Job drawing, mm, ordinate dimensions from the low corner. One solid piece. A direction names the side the tool comes from. Round coordinates to 2 decimals unless told otherwise and drop trailing zeros. Write each loop counter-clockwise with the first axis right and the second up, starting at its lowest first coordinate (ties: lowest second). Pieces come first, ordered by that corner, then holes.
1) Saw through at A-A (y = 180). Write the cut outline in (x, z), plus the area to 3 significant figures.
2) Which spindle directions (+Z, -Z, +X, -X, +Y, -Y) get a long thin tool onto all of the face, cutting with end or side? Do the marked faces 4, 5, 6 and 7. Say none if no direction does.
3) Saw through at B-B (z = 30). Write the cut outline in (x, y).
4) Saw through at D-D (z = 54). Write the cut outline in (x, y).
5) Wall check: probe 1 along Y at (x, z) = (17, 30); probe 2 along Y at (x, z) = (24, 30); probe 3 along Y at (x, z) = (42, 11). Give the ranges that are in metal, low to high.
6) Flat gauge pins, fed straight in: pin 1 (12.5 mm diameter, centred on x = 33.5, y = 165.5, fed in from +Z); pin 2 (8 mm diameter, centred on y = 51, z = 24, fed in from +X); pin 3 (1.5 mm diameter, centred on x = 47.5, z = 8, fed in from +Y). Where does each tip first touch, or does it go through?
7) Pull direction Y, two halves, no side cores. Call the marked faces 1, 2 and 3: +Y half, -Y half, draft (parallel to the pull), parting line (faces both ways), or undercut.
8) Saw through at C-C (y = 81). Write the cut outline in (x, z), plus the area to 3 significant figures.
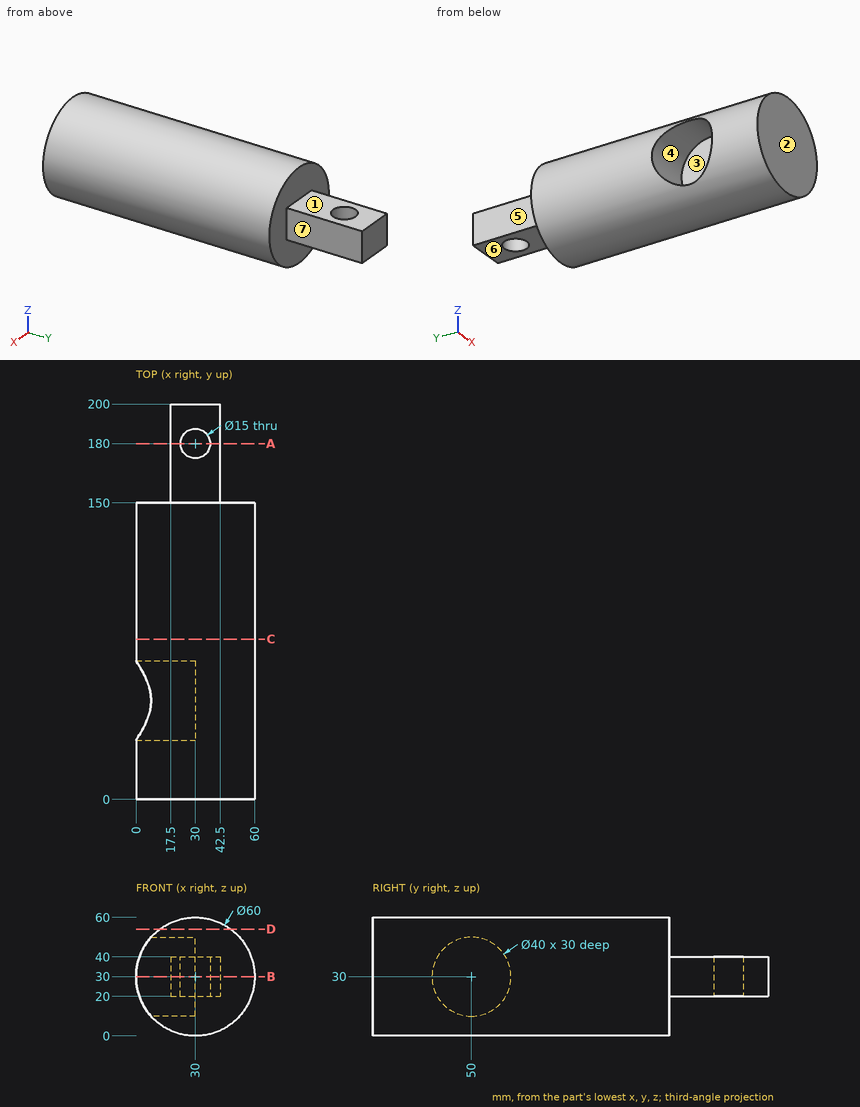
Evaluation:
1. outline: (17.5, 20) - (22.5, 20) - (22.5, 40) - (17.5, 40) - close; (37.5, 20) - (42.5, 20) - (42.5, 40) - (37.5, 40) - close
1. area: 200 mm2
2. face 4: -X
2. face 5: +Z, -Z, -X, +Y
2. face 6: -Z, +X, -X, +Y
2. face 7: +Z, -Z, +X, +Y
3. outline: (0, 0) - (60, 0) - (60, 150) - (42.5, 150) - (42.5, 200) - (17.5, 200) - (17.5, 150) - (0, 150) - (0, 70) - (30, 70) - (30, 30) - (0, 30) - close; hole circle Ø15 at (30, 180)
4. outline: (12, 0) - (48, 0) - (48, 150) - (12, 150) - close
5. probe 1: y = 0 to 30, 70 to 150
5. probe 2: y = 0 to 30, 70 to 175.5, 184.5 to 200
5. probe 3: y = 0 to 150
6. pin 1: stops at z = 40
6. pin 2: stops at x = 59.93
6. pin 3: stops at y = 150
7. face 1: draft
7. face 2: -Y half
7. face 3: undercut
8. outline: circle Ø60 at (30, 30)
8. area: 2,830 mm2
